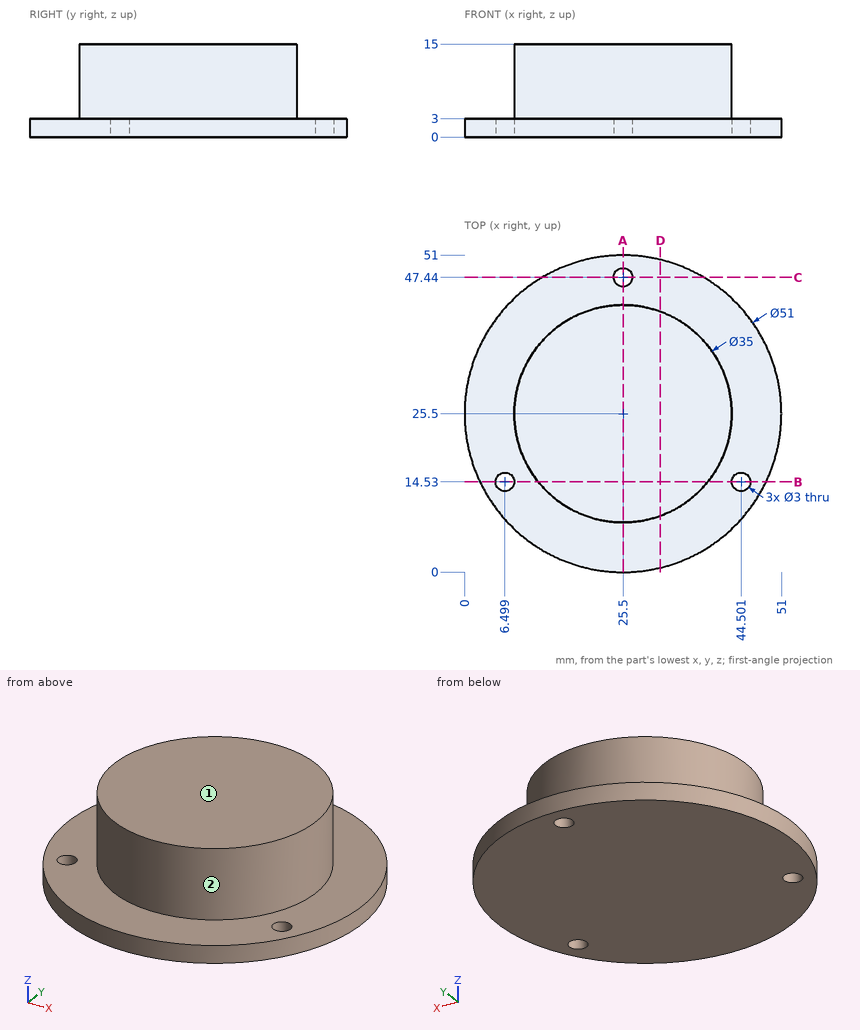
Source: three-view drawing plus pictorial views. Frame: mm from the lowest corner of the part. A direction names the side the tool comes from. Give positions to 0.01 mm unless a question says otherwise; leave off trailing zeros. Order: outer loops, then holes, each group sorted by start corner. A loop starts at its lowest first (then second) coordinate and runs counter-clockwise, first axis right, second up. Notation, with made-up numbers: (51.5, -38) -> (101.5, -38) arc R19 cw to (101.5, -31) -> close; hole circle Ø11 at (-3.5, 88.5). An arc over 180 degrees is marked (long way). Put each result on its own line as item: value.
Q1. Section A-A, the plane x = 25.5. Return loops of the section in (y, z).
Here are the results:
outline: (0, 0) -> (45.94, 0) -> (45.94, 3) -> (43, 3) -> (43, 15) -> (8, 15) -> (8, 3) -> (0, 3) -> close; (48.94, 0) -> (51, 0) -> (51, 3) -> (48.94, 3) -> close
Q2. Section B-B, the plane y = 14.53. Return loops of the section in (x, z) (1 decimal).
Here are the results:
outline: (2.5, 0) -> (5, 0) -> (5, 3) -> (2.5, 3) -> close; (8, 0) -> (43, 0) -> (43, 3) -> (39.1, 3) -> (39.1, 15) -> (11.9, 15) -> (11.9, 3) -> (8, 3) -> close; (46, 0) -> (48.5, 0) -> (48.5, 3) -> (46, 3) -> close
Q3. Section D-D, the plane x = 31.5. Return loops of the section in (y, z).
Here are the results:
outline: (0.72, 0) -> (50.28, 0) -> (50.28, 3) -> (41.94, 3) -> (41.94, 15) -> (9.06, 15) -> (9.06, 3) -> (0.72, 3) -> close
Q4. Material intervals for L1, parallel to X at y = 14.53, z = 0.8; L2, parallel to Y at x = 25.5, z = 1.45; L3, parallel to Z at x = 47.5, y = 35.5, sorted ascending.
Here are the results:
L1: x = 2.48 to 5, 8 to 43, 46 to 48.52
L2: y = 0 to 45.94, 48.94 to 51
L3: z = 0 to 3
Q5. Pin query (flat end, axial travel): pin 1 (8 mm diameter, centred on y = 32, z = 8, fed in from +X); pin 2 (2.5 mm diameter, centred on x = 44.5, y = 14.53, fed in from +Z); pin 3 (1.5 mm diameter, centred on x = 42.5, z = 2, fed in from +Y); pin 4 (5 mm diameter, centred on y = 16.5, z = 8.5, fed in from +X). Return the tip coordinate at first contact, or that it passes through.
Here are the results:
pin 1: stops at x = 42.82
pin 2: passes through
pin 3: stops at y = 45.15
pin 4: stops at x = 41.75
Q6. Reachability of the marked faces 1 and 2 from +Z, -Z, +X, -X, +Y, -Y: full face, straight path, thin tool, end or side. Return the list, or none.
Here are the results:
face 1: +Z, +X, -X, +Y, -Y
face 2: +Z
Q7. Section C-C, the plane y = 47.44. Return loops of the section in (x, z) (1 decimal).
Here are the results:
outline: (12.5, 0) -> (24, 0) -> (24, 3) -> (12.5, 3) -> close; (27, 0) -> (38.5, 0) -> (38.5, 3) -> (27, 3) -> close
